from build123d import *

# Parameters (mm, degrees)
BOSS_EXTRUDE1_DEPTH = 25
SKETCH2_R           = 3
BOSS_EXTRUDE2_DEPTH = 16.55
SKETCH3_R           = 3
CUT_EXTRUDE1_DEPTH  = 10
CHAMFER1_SIZE       = 0.5


with BuildPart() as part:
    # Sketch1 → Boss-Extrude1 (new body, symmetric)
    with BuildSketch(Plane.XY):
        Polygon((11, 7.65), (-11, 7.65), (-11, 6.25), (-4.75, 0), (4.75, 0), (11, 6.25), align=None)
    extrude(amount=BOSS_EXTRUDE1_DEPTH, both=True)

    # Sketch2 → Boss-Extrude2 (add)
    with BuildSketch(Plane(origin=(0, 7.65, 0), x_dir=(1, 0, 0), z_dir=(0, 1, 0))):
        Circle(SKETCH2_R)
    extrude(amount=BOSS_EXTRUDE2_DEPTH)

    # Sketch3 → Cut-Extrude1 (cut)
    with BuildSketch(Plane(origin=(0, 7.65, 0), x_dir=(1, 0, 0), z_dir=(0, 1, 0))):
        with Locations((0, 17.5)):
            Circle(SKETCH3_R)
        with Locations((0, -17.5)):
            Circle(SKETCH3_R)
    extrude(amount=-CUT_EXTRUDE1_DEPTH, mode=Mode.SUBTRACT)

    # Chamfer1
    chamfer1_edges = [part.edges().sort_by_distance(p)[0] for p in [
        (-3, 24.2, 0),
    ]]
    chamfer(chamfer1_edges, length=CHAMFER1_SIZE)


solid = part.part
Can you work these out from the model? Positions are in its coordinate system, mm. A direction names the side the tool comes from. Give positions to 0.01 mm unless a question says otherwise; leave off trailing zeros. Order: outer loops, then holes, each group sorted by start corner. A loop starts at its lowest first (then second) coordinate and runs counter-clockwise, first axis right, second up. Notation, with made-up numbers: M 58,79.25 L 112,79.25 A26 ccw 112,98.25 Z; hole C -31.5,12 d1. An arc over 180 degrees is marked long. Use one line per item in the form item = value. Start each with the question number.
Item 1: If we section it at A-A (x = 0): Write out the boundary of the cut face in (y, z).
Item 2: For faces 1 (the cylindrical face through (-3, 16, 0)), 2 (the flat face through (-11, 7, 0)), which set-ups out of +Z, -Z, +X, -X, +Y, -Y let a thin tool reach every point of the face, with its end or its side?
Item 3: Will these pins go through, and if not, where does the flat tip stop? pin 1 Ø8 at (y, z) = (16.5, -4.5) entering from +X; pin 2 Ø12 at (y, z) = (6, 19) entering from -X; pin 3 Ø2 at (x, z) = (6, 9.5) entering from -Y; pin 4 Ø1 at (x, z) = (-3, 10.5) entering from +Y.
Item 4: If we section it at B-B (z = 17.5): Write out the boundary of the cut face in (x, y).
Item 5: If I drill on line 1 along Z through (x, y) = (0, 3.25); line 2 along Y through (x, z) = (4.25, 2); line 3 along Z through (x, y) = (0.25, 22.5), over which ranges is the centre line in solid material (lowest first)?
Item 6: If we section it at D-D (y = 18.5): Write out the boundary of the cut face in (x, z).
Item 7: If we section it at C-C (z = 0): Write out the boundary of the cut face in (x, y).
Outcome:
q1.outline = M 0,-25 L 7.65,-25 L 7.65,-20.5 L 0,-20.5 Z; M 0,-14.5 L 7.65,-14.5 L 7.65,-3 L 23.7,-3 L 24.2,-2.5 L 24.2,2.5 L 23.7,3 L 7.65,3 L 7.65,14.5 L 0,14.5 Z; M 0,20.5 L 7.65,20.5 L 7.65,25 L 0,25 Z
q2.face_1 = +Y
q2.face_2 = +Z, -Z, -X, +Y, -Y
q3.pin_1 = 2.96
q3.pin_2 = -11
q3.pin_3 = 0.25
q3.pin_4 = 7.65
q4.outline = M -11,6.25 L -4.75,0 L -3,0 L -3,7.65 L -11,7.65 Z; M 3,0 L 4.75,0 L 11,6.25 L 11,7.65 L 3,7.65 Z
q5.line_1 = -25 to -20.5, -14.5 to 14.5, 20.5 to 25
q5.line_2 = 0 to 7.65
q5.line_3 = -2.99 to 2.99
q6.outline = C 0,0 d6
q7.outline = M -11,6.25 L -4.75,0 L 4.75,0 L 11,6.25 L 11,7.65 L 3,7.65 L 3,23.7 L 2.5,24.2 L -2.5,24.2 L -3,23.7 L -3,7.65 L -11,7.65 Z
